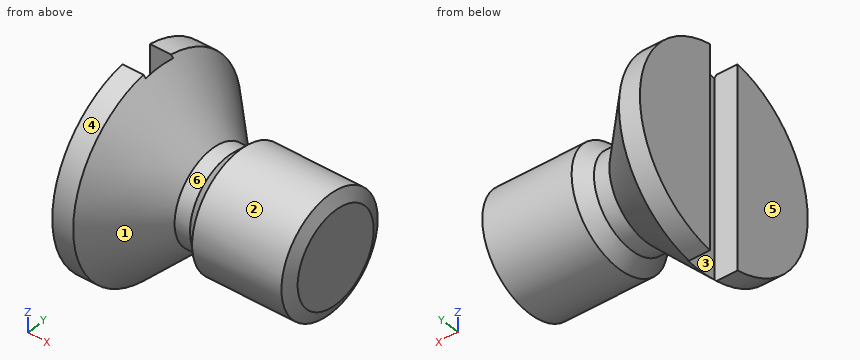
Autodesk Inventor part; units mm, degrees
ref_plane "Work Plane1" through (33.575, 0, 0) normal (0, 0, -1) x (1, 0, 0)
ref_plane "YZ Plane" through (0, 0, 0) normal (1, 0, 0) x (0, 1, 0)
ref_plane "XZ Plane" through (0, 0, 0) normal (0, 1, 0) x (-1, 0, 0)
sketch "Sketch1" plane through (0, 0, 0) normal (0, 0, 1) x (1, 0, 0)
  line L0 (0, 0) -> (6, 0)
  line L1 (6, 0) -> (6, 1.75)
  line L2 (6, 1.75) -> (3.13, 1.75)
  line L3 (3.13, 1.75) -> (2.7619, 1.3819)
  line L4 (2.7619, 1.3819) -> (2.2981, 1.3819)
  line L5 (2.2981, 1.3819) -> (0.63, 3.05)
  line L6 (0.63, 3.05) -> (0, 3.05)
  line L7 (0, 3.05) -> (0, 0)
  line L8 (3.13, 1.75) -> (1.93, 1.75) construction
  line L9 (-1.2, 0) -> (7.2, 0)
  line L10 (0, 3.66) -> (0, -0.61)
  dimension "d0" = 6
  dimension "d1" = 45
  dimension "d2" = 0.3681
  dimension "d3" = 2.87
  dimension "d4" = 1.93
  dimension "d5" = 2.7639
  dimension "d6" = 3.5
  dimension "d7" = 6.1
revolve "Body" add sketch "Sketch1" angle 360 about axis through (0, 0, 0) along (1, 0, 0)
sketch "Sketch2" plane through (0, 0, 0) normal (-1, 0, 0) x (0, 0, 1)
  line L0 (3.05, -0.5) -> (-3.05, -0.5)
  line L1 (-3.05, -0.5) -> (-3.05, 0.5)
  line L2 (-3.05, 0.5) -> (3.05, 0.5)
  line L3 (3.05, 0.5) -> (3.05, -0.5)
  line L4 (0, 0.5) -> (0, -0.5) construction
  line L5 (-3.05, 0) -> (3.05, 0) construction
  line L6 (0, 3.05) -> (0, 0)
  dimension "d15" = 1
  dimension "d16" = 6.1
extrude "Slot" cut sketch "Sketch2" against normal blind 0.7
thread "Thread"
chamfer "Chamfer1" distance 0.3681 distance2 0.184 1 edges at (6, -1.75, 0) measured on face at (6, 1.0235, -0.4633)
ref_plane "Work Plane1" through (33.575, 0, 0) normal (0, 0, -1) x (1, 0, 0)
equation "\"d0\" = NLG"
equation "\"d1\" = 0.5 * SEWI"
equation "\"d2\" = GAL"
equation "\"d3\" = GEL"
equation "\"d4\" = KOH"
equation "\"d5\" = BDM"
equation "\"d6\" = GD"
equation "\"d7\" = KOD"
equation "\"d15\" = SBR"
equation "\"d16\" = KOD"
equation "\"d8\" = STI"
equation "\"d10\" = GEL"
equation "\"d12\" = -0.5 * SPD + 0.5 * GD"
equation "\"d13\" = 0.5 * GAL"
equation "\"NLG\" = 6"
equation "\"GAL\" = 0.61345 * PTC"
equation "\"GEL\" = 2.87"
equation "\"KOH\" = 1.93"
equation "\"KOD\" = 6.1"
equation "\"SEWI\" = 90deg"
equation "\"BDM\" = NND - 1.2269 * PTC"
equation "\"GD\" = NND"
equation "\"SBR\" = 1"
equation "\"STI\" = 0.7"
equation "\"SPD\" = NND - 1.2269 * PTC"
equation "\"GUL\" = 0.61345 * PTC"
equation "\"PTC\" = 0.6"
equation "\"EPV\" = 3.68"
equation "\"THREADDIA\" = 3.5"
equation "\"TOA\" = 30deg"
equation "\"RR\" = 0.35"
equation "\"NND\" = 3.5"
equation "\"GD1\" = THREADDIA - 1.2269 * PTC"
properties part number "AS 1427 - M3.5 x 6" material "Steel, Mild"
Verification items for the finished model (mm, model axes). Face numbers are marked on the shaded views. A direction names the side the tool comes from. Coordinates: 2 decimals unless noted, no trailing zeros. Write each loop counter-clockwise with the first axis right and the second up, starting at its lowest first coordinate (ties: lowest second). Pieces come first, ordered by that corner, then holes. Notation, with made-up numbers: (57.25, 12.5) -> (98.25, 12.5) arc R32 ccw to (98.25, 40.5) -> close; hole circle Ø6 at (47, -13). An arc over 180 degrees is marked (long way). One line per item, written item: value. Start each with the question number.
Q1. Cross-section at A-A on z = 0. Enter the section's corners in (x, y), and give its area (3 significant figures).
Q2. Cross-section at B-B on y = 0. Enter the section's corners in (x, z).
Q3. Go/stop test with flat-tipped pins: P1, Ø2, axis at x = 1.5, y = 2, coming from the +Z side; P2, Ø0.8, axis at x = 0.5, z = -1, coming from the +Y side; P3, Ø1, axis at x = 3.5, y = -1.5, coming from the -Z side. Record where each tip stops, or that it passes through.
Q4. Access from +Z, -Z, +X, -X, +Y, -Y to the whole of each face (thin tool, end or side, straight path). Record for the marked faces 1, 2 and 3.
Q5. Cross-section at D-D on x = 5.25. Enter the section's corners in (y, z), and give its area (3 significant figures).
Q6. Thickness scan on L1, parallel to Z at x = 5.5, y = -1.5; L2, parallel to Y at x = 2.5, z = 0.75; L3, parallel to Z at x = 3, y = -0.25. Record the ranges inside material, lowest first. Write a range as from..to.
Q7. Cross-section at C-C on x = 1.25. Enter the section's corners in (y, z), and give its area (3 significant figures).
Q8. Mould release check, pull along X, two halves, no side actions. Record for the marked faces 4, 5 and 6: pulls with the +X half, pulls with the -X half, needs draft (parallel to the pull), parting line crosses it, or undercut.
Checked values:
1. outline: (0, -3.05) -> (0.63, -3.05) -> (2.3, -1.38) -> (2.76, -1.38) -> (3.13, -1.75) -> (5.82, -1.75) -> (6, -1.38) -> (6, 1.38) -> (5.82, 1.75) -> (3.13, 1.75) -> (2.76, 1.38) -> (2.3, 1.38) -> (0.63, 3.05) -> (0, 3.05) -> (0, 0.5) -> (0.7, 0.5) -> (0.7, -0.5) -> (0, -0.5) -> close
1. area: 22.9 mm²
2. outline: (0.7, -2.98) -> (2.3, -1.38) -> (2.76, -1.38) -> (3.13, -1.75) -> (5.82, -1.75) -> (6, -1.38) -> (6, 1.38) -> (5.82, 1.75) -> (3.13, 1.75) -> (2.76, 1.38) -> (2.3, 1.38) -> (0.7, 2.98) -> close
3. P1: stops at z = 2.65
3. P2: stops at y = 2.99
3. P3: stops at z = -1.44
4. face 1: none
4. face 2: +X
4. face 3: +Z, -Z, -X
5. outline: circle Ø3.5 at (0, 0)
5. area: 9.62 mm²
6. L1: z = -0.9..0.9
6. L2: y = -1.16..1.16
6. L3: z = -1.6..1.6
7. outline: circle Ø4.86 at (0, 0)
7. area: 18.6 mm²
8. face 4: needs draft
8. face 5: pulls with the -X half
8. face 6: undercut
